Autodesk Inventor part; units mm, degrees
ref_plane "YZ Plane" through (0, 0, 0) normal (1, 0, 0) x (0, 1, 0)
ref_plane "XZ Plane" through (0, 0, 0) normal (0, 1, 0) x (-1, 0, 0)
ref_plane "XY Plane" through (0, 0, 0) normal (0, 0, 1) x (1, 0, 0)
sketch "Sketch1" plane through (0, 0, 0) normal (0, 0, 1) x (1, 0, 0)
  line L0 (0, 0) -> (12.3503, 0)
  line L1 (12.3503, 0) -> (12.3503, 19)
  line L2 (12.3503, 19) -> (0, 19)
  line L3 (0, 19) -> (0, 0)
  line L4 (0, 19) -> (25.485, 19)
  line L5 (25.485, 19) -> (25.485, 22.5)
  line L6 (25.485, 22.5) -> (0, 22.5)
  line L7 (0, 22.5) -> (0, 19)
  line L8 (23.226, 22.5) -> (23.226, 25.5)
  line L9 (23.226, 25.5) -> (0, 25.5)
  line L10 (0, 25.5) -> (0, 22.5)
  line L11 (23.226, 25.5) -> (25.485, 25.5)
  line L12 (25.485, 25.5) -> (25.485, 33.5)
  line L13 (25.485, 33.5) -> (20.485, 33.5)
  line L14 (20.485, 33.5) -> (20.485, 22.5)
  dimension "d0" = 19
  dimension "d1" = 25.485
  dimension "d2" = 3.5
  dimension "d3" = 90
  dimension "d4" = 3
  dimension "d5" = 8
  dimension "d6" = 5
revolve "Revolution1" add sketch "Sketch1" angle 360 about axis through (0, 19, 0) along (0, -1, 0)
sketch "Sketch2" plane through (0, 33.5, 0) normal (0, 1, 0) x (1, 0, 0)
  line L0 (25.0712, -4.4185) -> (24.0712, -4.4185)
  line L1 (24.0712, -4.4185) -> (24.0712, 4.5815)
  line L2 (24.0712, 4.5815) -> (25.0712, 4.5815)
  line L3 (25.0712, 4.5815) -> (25.0712, -4.4185)
  line L4 (-23.9768, -4.4185) -> (-24.9768, -4.4185)
  line L5 (-24.9768, -4.4185) -> (-24.9768, 4.5815)
  line L6 (-24.9768, 4.5815) -> (-23.9768, 4.5815)
  line L7 (-23.9768, 4.5815) -> (-23.9768, -4.4185)
  point P0 (0, 0)
  dimension "d8" = 1
  dimension "d9" = 9
  dimension "d10" = 1
  dimension "d11" = 9
extrude "Extrusion1" add sketch "Sketch2" along normal blind 60
sketch "Sketch3" plane through (0, 93.5, 0) normal (0, 1, 0) x (1, 0, 0)
  circle A0 centre (0, 0) radius 12.3503
  circle A1 centre (0, 0) radius 25.485
extrude "Extrusion2" add sketch "Sketch3" along normal blind 10
sketch "Sketch4" plane through (0, 103.5, 0) normal (0, 1, 0) x (1, 0, 0)
  point P0 (0, 0)
sketch "Sketch5" plane through (0, 103.5, 0) normal (0, 1, 0) x (1, 0, 0)
  circle A0 centre (0, 0) radius 24.5
  dimension "d16" = 49
extrude "Extrusion3" add sketch "Sketch5" along normal blind 49
fillet "Fillet1" radius 10 1 edges at (-24.5, 152.5, 0)
sketch "Sketch6" plane through (-23.9768, 33.5, 4.4185) normal (1, 0, 0) x (0, 0, -1)
  line L0 (0, 0) -> (0, 60)
  line L1 (9, 0) -> (9, 60)
  line L2 (0, 19.4645) -> (9, 19.4645)
  line L3 (9, 19.4645) -> (9, 46.9149)
  line L4 (9, 46.9149) -> (0, 46.9149)
  line L5 (0, 46.9149) -> (0, 19.4645)
  point P0 (4.4185, -33.5)
extrude "Extrusion4" add sketch "Sketch6" along normal blind 49
thread "Thread1"
properties part number "Part 3 of Focusrite Microphone"
For this review, take the finished solid that the model builds, in its own axes (mm). A direction names the side the tool comes from. Round coordinates to 2 decimals unless told otherwise and drop trailing zeros. Write each loop counter-clockwise with the first axis right and the second up, starting at its lowest first coordinate (ties: lowest second). Pieces come first, ordered by that corner, then holes. Notation, with made-up numbers: (55, 62.25) -> (80, 62.25) arc R17 cw to (80, 80.25) -> close; hole circle Ø5 at (11, 40). An arc over 180 degrees is marked (long way). Use one line per item in the form item = value.
Q1. To check wall thickness, follow probe 1 along Y at (x, z) = (12.5, 0.5); probe 2 along Y at (x, z) = (20.5, 15); probe 3 along X at (y, z) = (98, 0) (3 decimals). State the ranges of each line that lie inside material, in increasing order. Write a range as from..to.
Resolved:
probe_1 = 19..25.5, 52.96..80.41, 93.5..152.5
probe_2 = 19..22.5, 25.5..33.5, 93.5..103.5
probe_3 = -25.485..-12.35, 12.35..25.485
Q2. The part is to be moulded in two halves that separate along Y. For faces 6 (the flat face through (0, 152.5, 0)), 7 (the flat face through (-24.977, 63, 0)), 8 (the cylindrical face through (13.17, 122.73, 20.66)), 9 (the flat face through (0, 0, 0)), say which applies: released by +Y, released by -Y, zero draft, split by the parting line, or undercut.
Resolved:
face_6 = released by +Y
face_7 = undercut
face_8 = zero draft
face_9 = released by -Y
Q3. Machinability: for faces 1 (the flat face through (-13, 103.5, -21)), 2 (the flat face through (-23.977, 43, 0)), 3 (the cylindrical face through (-20.22, 29.56, 15.51)), 4 (the cylindrical face through (-9.801, 9.633, 7.515)), 5 (the flat face through (23, 22.5, 6)), which of the approach directions +Z, -Z, +X, -X, +Y, -Y give a long, thin tool a straight path to every point of the face, cutting with its end or side? Answer none if there is none.
Resolved:
face_1 = +Y
face_2 = +Z, -Z
face_3 = +Y, -Y
face_4 = -Y
face_5 = none
Q4. Consider section B-B (x = 0). State how many separate pieces and enclosed holes the cut face has, then the cut area to 3 significant figures.
Resolved:
separate_pieces = 3
enclosed_holes = 0
area = 3,730 mm²
Q5. Consider section C-C (y = 67.5). State the section outline as (x, z) points, then the cut area to 3 significant figures.
Resolved:
outline = (-24.98, -4.58) -> (25.07, -4.58) -> (25.07, 4.42) -> (-24.98, 4.42) -> close
area = 450 mm²
Q6. Consider section A-A (y = 44). State the section outline as (x, z) points.
Resolved:
outline = (-24.98, -4.58) -> (-23.98, -4.58) -> (-23.98, 4.42) -> (-24.98, 4.42) -> close; (24.07, -4.58) -> (25.07, -4.58) -> (25.07, 4.42) -> (24.07, 4.42) -> close
Q7. Clearance check with flat-ended pins moving along their axes: pin 1 Ø7 at (y, z) = (60.5, 0.5) entering from +X; pin 2 Ø5 at (x, y) = (10.5, 131.5) entering from -Z; pin 3 Ø6 at (x, y) = (-17, 34.5) entering from +Z. State where each tip first meets the part, or that it passes through.
Resolved:
pin_1 = 25.07
pin_2 = -23.16
pin_3 = 21.18
